The model under review builds one solid part; all positions refer to its coordinate system, in mm. A direction names the side the tool comes from. Give positions to 0.01 mm unless a question says otherwise; leave off trailing zeros. Order: outer loops, then holes, each group sorted by start corner. A loop starts at its lowest first (then second) coordinate and runs counter-clockwise, first axis right, second up. Notation, with made-up numbers: (62.25, 4) - (83.25, 4) arc R22 cw to (83.25, 39) - close; hole circle Ø3 at (-25, -27.75). An arc over 180 degrees is marked (long way). Use a Markdown table: item, result. Add a question column.
```python
from build123d import *

# Parameters (mm, degrees)
SKETCH1_R           = 3
BOSS_EXTRUDE1_DEPTH = 40
SKETCH2_R           = 1.5
CUT_EXTRUDE1_DEPTH  = 20
SKETCH6_W           = 80
SKETCH6_H           = 4
CUT_EXTRUDE4_DEPTH  = 15
FILLET1_R           = 10
FILLET2_R           = 5
FILLET3_R           = 2
SKETCH7_R           = 6
CUT_EXTRUDE5_DEPTH  = 5


with BuildPart() as part:
    # Sketch1 → Boss-Extrude1 (new body)
    with BuildSketch(Plane.XY):
        Polygon((40, 0), (-40, 0), (-40, -8), (-9.545454545, -8), (-9.545454545, -23), (9.545454545, -23), (9.545454545, -8), (40, -8), align=None)
        with Locations((0, -15)):
            Circle(SKETCH1_R, mode=Mode.SUBTRACT)
    extrude(amount=BOSS_EXTRUDE1_DEPTH)

    # Sketch2 → Cut-Extrude1 (cut)
    with BuildSketch(Plane(origin=(0, 0, 0), x_dir=(-1, 0, 0), z_dir=(0, 0, -1))):
        with Locations((32, -4)):
            Circle(SKETCH2_R)
    extrude(amount=-CUT_EXTRUDE1_DEPTH, mode=Mode.SUBTRACT)

    # Sketch6 → Cut-Extrude4 (cut)
    with BuildSketch(Plane.XZ.offset(23)):
        with Locations((0, 20)):
            Rectangle(SKETCH6_W, SKETCH6_H)
    extrude(amount=-CUT_EXTRUDE4_DEPTH, mode=Mode.SUBTRACT)

    # Fillet1
    # the kernel refuses this fillet: 10 mm, written as the material it takes off along each edge
    with BuildSketch(Plane(origin=(40, -33, 40), x_dir=(-1, 0, 0), z_dir=(0, 1, 0)), Plane(origin=(-40, 25, 40), x_dir=(1, 0, 0), z_dir=(0, -1, 0))) as fillet1_piece_1:
        with BuildLine():
            CenterArc((FILLET1_R, -FILLET1_R), FILLET1_R, 90, 90)
            Line((0, -FILLET1_R), (0, 0))
            Line((0, 0), (FILLET1_R, 0))
        make_face()
    extrude(amount=58, mode=Mode.SUBTRACT)
    with BuildSketch(Plane(origin=(-40, 25, 0), x_dir=(1, 0, 0), z_dir=(0, -1, 0)), Plane(origin=(40, -33, 0), x_dir=(-1, 0, 0), z_dir=(0, 1, 0))) as fillet1_piece_2:
        with BuildLine():
            CenterArc((FILLET1_R, FILLET1_R), FILLET1_R, 180, 90)
            Line((0, FILLET1_R), (0, 0))
            Line((0, 0), (FILLET1_R, 0))
        make_face()
    extrude(amount=58, mode=Mode.SUBTRACT)

    # Fillet2
    fillet2_edges = [part.edges().sort_by_distance(p)[0] for p in [
        (9.545454545, -23, 31),
        (-9.545454545, -23, 31),
        (9.545454545, -23, 9),
        (-9.545454545, -23, 9),
    ]]
    fillet(fillet2_edges, radius=FILLET2_R)

    # Fillet3
    fillet3_edges = [part.edges().sort_by_distance(p)[0] for p in [
        (9.545454545, -8, 31),
        (-9.545454545, -8, 31),
        (9.545454545, -8, 9),
        (-9.545454545, -8, 9),
    ]]
    fillet(fillet3_edges, radius=FILLET3_R)

    # Sketch7 → Cut-Extrude5 (cut)
    with BuildSketch(Plane(origin=(0, 0, 0), x_dir=(1, 0, 0), z_dir=(0, 1, 0))):
        with Locations(Location((0, -20, 0), (0, 0, 180))):
            Circle(SKETCH7_R)
    extrude(amount=-CUT_EXTRUDE5_DEPTH, mode=Mode.SUBTRACT)


solid = part.part
```
Q1. We need section B-B (z = 4). Write out the cut boundary in (x, y), plus the area to 3 significant figures.
Q2. Draft analysis for pull direction Z (two halves, no side actions). For faces 4 (the cylindrical face through (36.99, -4.06, 37.15)), 5 (the cylindrical face through (-0.65, -17.93, 30.87)), 6 (the flat face through (0, -5, 20)), state which applies: pulls with the +Z half, pulls with the -Z half, needs draft (parallel to the pull), parting line crosses it, or undercut.
Q3. Wall thickness on probe 1 along Z at (x, y) = (5, -12.5); probe 2 along Y at (x, z) = (-32, 14); probe 3 along Z at (x, y) = (0, -1.7): over which ranges is each line inside the solid? List them lowest first.
Q4. Machinability: for faces 1 (the flat face through (-9.545, -14, 9)), 2 (the flat face through (-3, -17, 18)), 3 (the cylindrical face through (-30.5, -3.93, 9.87)), which of the approach directions +Z, -Z, +X, -X, +Y, -Y give a long, thin tool a straight path to every point of the face, cutting with its end or side? Answer none if there is none.
Q5. Clearance check with flat-ended pins moving along their axes: P1, Ø6.5, axis at y = -14.5, z = 8, coming from the +X side; P2, Ø1, axis at y = -11, z = 27, coming from the -X side; P3, Ø3, axis at x = 1, z = 16.5, coming from the +Y side. State where each tip first meets the part, or that it passes through.
Q6. We need section C-C (x = 0). Write out the cut boundary in (y, z), plus the area to 3 significant figures.
Q7. We need section A-A (y = -15). Write out the cut boundary in (x, z), plus the area to 3 significant figures.
Q8. We need section D-D (y = -4). Write out the cut boundary in (x, z), plus the area to 3 significant figures.
Here are the results:
| question | item | result |
|---|---|---|
| 1 | outline | (-38, -8) - (-11.55, -8) arc R2 cw to (-9.55, -10) - (-9.55, -18) arc R5 ccw to (-4.55, -23) - (4.55, -23) arc R5 ccw to (9.55, -18) - (9.55, -10) arc R2 cw to (11.55, -8) - (38, -8) - (38, 0) - (-38, 0) - close; hole circle Ø3 at (-32, -4); hole circle Ø6 at (0, -15) |
| 1 | area | 850 mm2 |
| 2 | face 4 | pulls with the +Z half |
| 2 | face 5 | needs draft |
| 2 | face 6 | undercut |
| 3 | probe 1 | 0 to 18, 22 to 40 |
| 3 | probe 2 | -8 to -5.5, -2.5 to 0 |
| 3 | probe 3 | 0 to 14, 26 to 40 |
| 4 | face 1 | +Z, -Z, -X, -Y |
| 4 | face 2 | +X, -X, -Y |
| 4 | face 3 | -Z |
| 5 | P1 | x = 9.55 |
| 5 | P2 | x = -9.55 |
| 5 | P3 | y = -5 |
| 6 | outline | (-23, 0) - (-18, 0) - (-18, 18) - (-23, 18) - close; (-23, 22) - (-18, 22) - (-18, 40) - (-23, 40) - close; (-12, 0) - (0, 0) - (0, 14) - (-5, 14) - (-5, 26) - (0, 26) - (0, 40) - (-12, 40) - (-12, 22) - (-8, 22) - (-8, 18) - (-12, 18) - close |
| 6 | area | 584 mm2 |
| 7 | outline | (-9.55, 0) - (-3, 0) - (-3, 18) - (-9.55, 18) - close; (-9.55, 22) - (-3, 22) - (-3, 40) - (-9.55, 40) - close; (3, 0) - (9.55, 0) - (9.55, 18) - (3, 18) - close; (3, 22) - (9.55, 22) - (9.55, 40) - (3, 40) - close |
| 7 | area | 471 mm2 |
| 8 | outline | (-40, 10) arc R10 ccw to (-33.5, 0.63) - (-33.5, 20) - (-30.5, 20) - (-30.5, 0.01) arc R10 ccw to (-30, 0) - (30, 0) arc R10 ccw to (40, 10) - (40, 30) arc R10 ccw to (30, 40) - (-30, 40) arc R10 ccw to (-40, 30) - close; hole circle Ø12 at (0, 20) |
| 8 | area | 2,940 mm2 |
